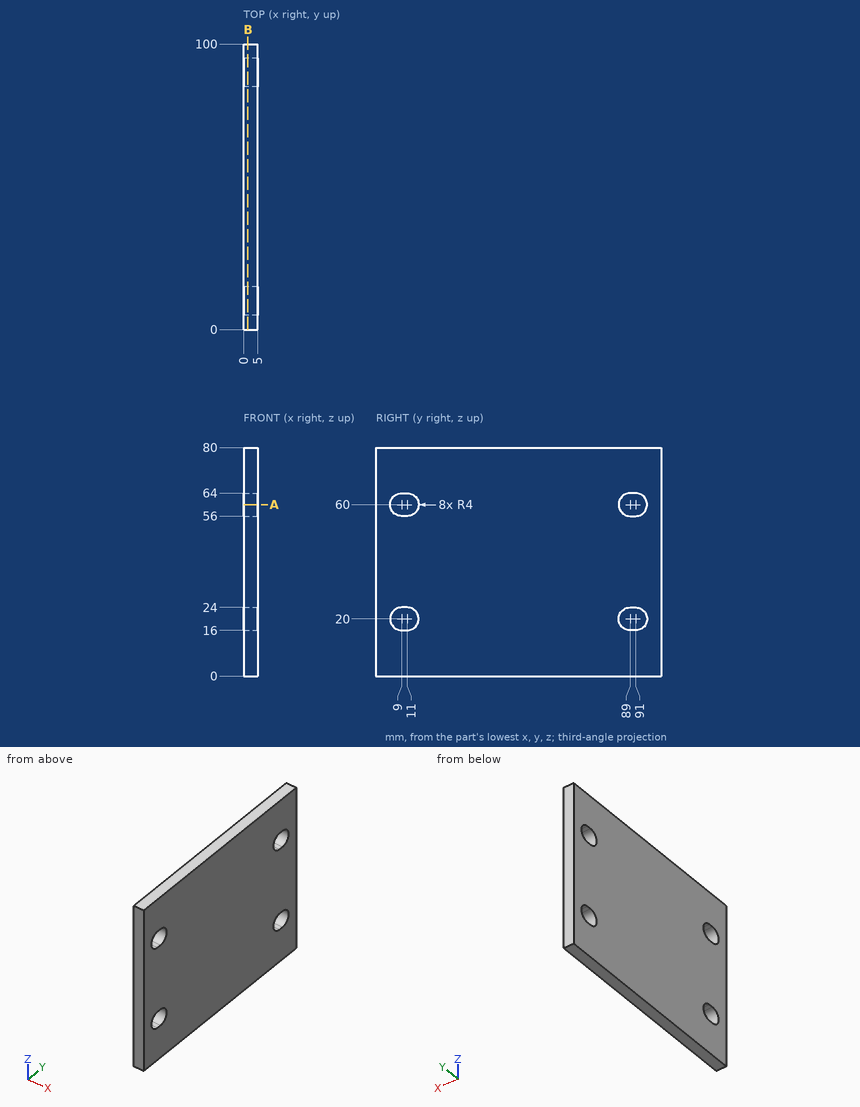
Check sheet for the drawn part. Datum: minimum x, y, z corner. Units: mm. Coordinates: 2 decimals unless noted, no trailing zeros. Loops run counter-clockwise (first coordinate to the right, second up) from the corner with the lowest first, then second, coordinate; pieces in that order, holes last. Notation, with made-up numbers: (-28.5, 50) -> (-21.5, 50) arc R11 ccw to (-21.5, 59) -> close; hole circle Ø5 at (54.25, 37). An arc over 180 degrees is marked (long way). Answer as CSV lines item,"result".
1) Thickness scan on L1, parallel to Y at x = 3.2, z = 20; L2, parallel to Y at x = 0.6, z = 56.5; L3, parallel to Z at x = 0.65, y = 14. Record the ranges inside material, lowest first. Write a range as from..to.
Found:
L1,"y = 0..5, 15..85, 95..100"
L2,"y = 0..7.06, 12.94..87.06, 92.94..100"
L3,"z = 0..17.35, 22.65..57.35, 62.65..80"
2) Cross-section at A-A, the plane z = 60. Record the cut outline in (x, y).
Found:
outline,"(0, 0) -> (5, 0) -> (5, 5) -> (0, 5) -> close; (0, 15) -> (5, 15) -> (5, 85) -> (0, 85) -> close; (0, 95) -> (5, 95) -> (5, 100) -> (0, 100) -> close"
3) Cross-section at B-B, the plane x = 1.5. Record the cut outline in (y, z), then the cut area to 3 significant figures.
Found:
outline,"(0, 0) -> (100, 0) -> (100, 80) -> (0, 80) -> close; hole (9, 16) -> (11, 16) arc R4 ccw to (11, 24) -> (9, 24) arc R4 ccw to start; hole (9, 56) -> (11, 56) arc R4 ccw to (11, 64) -> (9, 64) arc R4 ccw to start; hole (89, 16) -> (91, 16) arc R4 ccw to (91, 24) -> (89, 24) arc R4 ccw to start; hole (89, 56) -> (91, 56) arc R4 ccw to (91, 64) -> (89, 64) arc R4 ccw to start"
area,"7,730 mm2"
